Verification items for the finished model (mm, model axes). Give positions to 0.01 mm unless a question says otherwise; leave off trailing zeros. Order: outer loops, then holes, each group sorted by start corner. A loop starts at its lowest first (then second) coordinate and runs counter-clockwise, first axis right, second up.
from build123d import *

# Parameters (mm, degrees)
SKETCH_1_R          = 8
EXTRUDE_1_DEPTH     = 24
SKETCH_2_R          = 42
EXTRUDE_2_DEPTH     = 18
SKETCH_4_OUTSIDE_W  = 110.238
SKETCH_4_OUTSIDE_H  = 110.238
SKETCH_4_OUTSIDE_R  = 5.1
CUT_EXTRUDE_2_DEPTH = 65.062469512


with BuildPart() as part:
    # 草图1 → 凸台-拉伸1 (new body)
    with BuildSketch(Plane.XY):
        Circle(SKETCH_1_R)
    extrude(amount=EXTRUDE_1_DEPTH)

    # 草图2 → 凸台-拉伸2 (add)
    with BuildSketch(Plane.XY):
        Circle(SKETCH_2_R)
    extrude(amount=EXTRUDE_2_DEPTH)

    # 草图4 outside → 切除-拉伸2 (cut, through all)
    with BuildSketch(Plane.XY.offset(24)):
        Rectangle(SKETCH_4_OUTSIDE_W, SKETCH_4_OUTSIDE_H)
        Circle(SKETCH_4_OUTSIDE_R, mode=Mode.SUBTRACT)
    extrude(amount=-CUT_EXTRUDE_2_DEPTH, mode=Mode.SUBTRACT)


solid = part.part
(1) Scan lines: line 1 (X direction, y = 0.25, z = 20.5); line 2 (Y direction, x = 1, z = 11.5); line 3 (Y direction, x = -3, z = 2). Record each from-to range of solid material in increasing order.
Solved:
line 1: x = -5.09 to 5.09
line 2: y = -5 to 5
line 3: y = -4.12 to 4.12
(2) Go/stop test with flat-tipped pins: pin 1 (5 mm diameter, centred on x = -3, z = 6.5, fed in from +Y); pin 2 (1 mm diameter, centred on y = -1, z = 3, fed in from -X); pin 3 (1 mm diameter, centred on y = -2, z = 20.5, fed in from -X). Record where each tip stops, or that it passes through.
Solved:
pin 1: stops at y = 5.08
pin 2: stops at x = -5.08
pin 3: stops at x = -4.87
(3) Section check B-B, the plane x = 2. Enter the section's corners in (y, z), then the cut area to 3 significant figures.
Solved:
outline: (-4.69, 0) - (4.69, 0) - (4.69, 24) - (-4.69, 24) - close
area: 225 mm2
(4) Section check A-A, the plane z = 13. Enter the section's corners in (x, y).
Solved:
outline: circle Ø10.2 at (0, 0)
(5) Section check C-C, the plane y = -3.5. Enter the section's corners in (x, z), then the cut area to 3 significant figures.
Solved:
outline: (-3.71, 0) - (3.71, 0) - (3.71, 24) - (-3.71, 24) - close
area: 178 mm2
